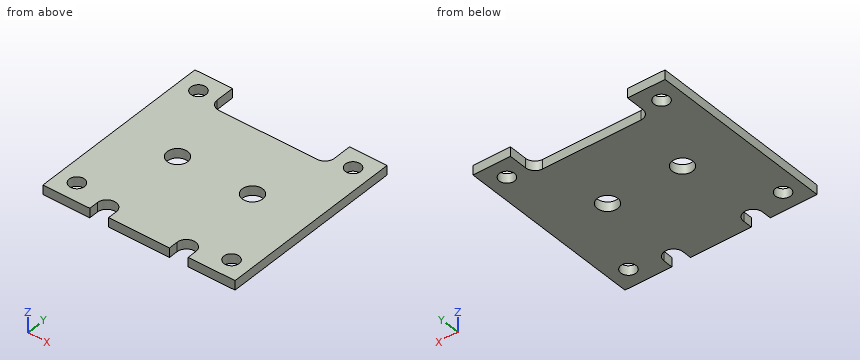
```python
from build123d import *

# Parameters (mm, degrees)
SKETCH1_W               = 130.175
SKETCH1_H               = 127
EXTRUDE1_DEPTH          = 6.35
F_3_8_CLEARANCE_HOLE1_D = 10.31748
SKETCH4_W               = 79.375
SKETCH4_H               = 19.05
EXTRUDE2_DEPTH          = 92.153470347
FILLET2_R               = 6.35
SKETCH5_W               = 12.7
SKETCH5_H               = 6.35
EXTRUDE3_DEPTH          = 92.153470347
SKETCH6_R               = 6.35
EXTRUDE4_DEPTH          = 92.153470347
F_1_2_CLEARANCE_HOLE1_D = 13.89126


with BuildPart() as part:
    # Sketch1 → Extrude1 (new body)
    with BuildSketch(Plane.XY):
        Rectangle(SKETCH1_W, SKETCH1_H)
    extrude(amount=-EXTRUDE1_DEPTH)

    # 3/8 Clearance Hole1 (through all)
    with Locations(Plane.XY):
        with Locations((-52.3875, 50.8), (52.3875, 50.8), (52.3875, -50.8), (-52.3875, -50.8)):
            Hole(F_3_8_CLEARANCE_HOLE1_D / 2)

    # Sketch4 → Extrude2 (cut, through all)
    with BuildSketch(Plane.XY):
        with Locations((0, 53.975)):
            Rectangle(SKETCH4_W, SKETCH4_H)
    extrude(amount=-EXTRUDE2_DEPTH, mode=Mode.SUBTRACT)

    # Fillet2
    fillet2_edges = [part.edges().sort_by_distance(p)[0] for p in [
        (-39.6875, 44.45, -3.175),
        (39.6875, 44.45, -3.175),
    ]]
    fillet(fillet2_edges, radius=FILLET2_R)

    # Sketch5 → Extrude3 (cut, through all)
    with BuildSketch(Plane(origin=(0, 0, -6.35), x_dir=(-1, 0, 0), z_dir=(0, 0, -1))):
        with Locations((-26.9875, -60.325)):
            Rectangle(SKETCH5_W, SKETCH5_H)
    extrude3 = extrude(amount=-EXTRUDE3_DEPTH, mode=Mode.SUBTRACT)

    # Sketch6 → Extrude4 (cut, through all)
    with BuildSketch(Plane(origin=(0, 0, -6.35), x_dir=(-1, 0, 0), z_dir=(0, 0, -1))):
        with Locations((-26.9875, -57.15)):
            Circle(SKETCH6_R)
    extrude4 = extrude(amount=-EXTRUDE4_DEPTH, mode=Mode.SUBTRACT)

    # Mirror2: Extrude3, Extrude4 across plane
    add(extrude3.mirror(Plane(origin=(0, 0, 0), x_dir=(0, 0, 1), z_dir=(1, 0, 0))), mode=Mode.SUBTRACT)
    add(extrude4.mirror(Plane(origin=(0, 0, 0), x_dir=(0, 0, 1), z_dir=(1, 0, 0))), mode=Mode.SUBTRACT)

    # 1/2 Clearance Hole1 (through all)
    with Locations(Plane(origin=(0, 0, -6.35), x_dir=(-1, 0, 0), z_dir=(0, 0, -1))):
        with Locations((-25.4, 0), (25.4, 0)):
            Hole(F_1_2_CLEARANCE_HOLE1_D / 2)


solid = part.part
```
Model file for the job. Use its own axes, mm. Give positions to 0.01 mm unless a question says otherwise; leave off trailing zeros. Loops run counter-clockwise (first coordinate to the right, second up) from the corner with the lowest first, then second, coordinate; pieces in that order, holes last. Notation, with made-up numbers: (59.5, 26) -> (99.5, 26) arc R22 cw to (99.5, 49) -> close; hole circle Ø11 at (24, 19). An arc over 180 degrees is marked (long way). Use CSV: the item, a comma, the result in double quotes. Start each with the question number.
1) Flat gauge pin, fed straight in: pin 1 Ø9.5 at (x, y) = (52.39, 50.8) entering from +Z. Where does the tip first touch, or does it go through?
2) Slice it at A-A on y = 0. Give the cut face in (x, z), plus the area to 3 significant figures.
3) Slice it at B-B on z = -3.5. Give the cut face in (x, y).
4) Wall check: line 1 (Y direction, x = 34, z = -2); line 2 (Y direction, x = -56.5, z = -3.25); line 3 (Y direction, x = 28.5, z = -2). Give the ranges that are in metal, low to high.
5) Slice it at D-D on x = 4.5. Give the cut face in (y, z), plus the area to 3 significant figures.
6) Slice it at C-C on x = -25.4. Give the cut face in (y, z), plus the area to 3 significant figures.
Computed values:
1,pin 1,"passes through"
2,outline,"(-65.09, -6.35) -> (-32.35, -6.35) -> (-32.35, 0) -> (-65.09, 0) -> close; (-18.45, -6.35) -> (18.45, -6.35) -> (18.45, 0) -> (-18.45, 0) -> close; (32.35, -6.35) -> (65.09, -6.35) -> (65.09, 0) -> (32.35, 0) -> close"
2,area,"650 mm^2"
3,outline,"(-65.09, -63.5) -> (-33.34, -63.5) -> (-33.34, -57.15) arc R6.35 cw to (-20.64, -57.15) -> (-20.64, -63.5) -> (20.64, -63.5) -> (20.64, -57.15) arc R6.35 cw to (33.34, -57.15) -> (33.34, -63.5) -> (65.09, -63.5) -> (65.09, 63.5) -> (39.69, 63.5) -> (39.69, 50.8) arc R6.35 cw to (33.34, 44.45) -> (-33.34, 44.45) arc R6.35 cw to (-39.69, 50.8) -> (-39.69, 63.5) -> (-65.09, 63.5) -> close; hole circle Ø10.32 at (-52.39, -50.8); hole circle Ø10.32 at (-52.39, 50.8); hole circle Ø13.89 at (-25.4, 0); hole circle Ø13.89 at (25.4, 0); hole circle Ø10.32 at (52.39, -50.8); hole circle Ø10.32 at (52.39, 50.8)"
4,line 1,"y = -63.5 to 44.48"
4,line 2,"y = -63.5 to -53.91, -47.69 to 47.69, 53.91 to 63.5"
4,line 3,"y = -50.98 to -6.22, 6.22 to 44.45"
5,outline,"(-63.5, -6.35) -> (44.45, -6.35) -> (44.45, 0) -> (-63.5, 0) -> close"
5,area,"685 mm^2"
6,outline,"(-51, -6.35) -> (-6.95, -6.35) -> (-6.95, 0) -> (-51, 0) -> close; (6.95, -6.35) -> (44.45, -6.35) -> (44.45, 0) -> (6.95, 0) -> close"
6,area,"518 mm^2"
